```python
from build123d import *
from OCP.BRepFilletAPI import BRepFilletAPI_MakeChamfer

# Parameters (mm, degrees)
BOSS_EXTRUDE1_DEPTH = 20
SKETCH4_W           = 1
SKETCH4_H           = 9
CUT_EXTRUDE2_DEPTH  = 20
CUT_EXTRUDE4_START  = -2
CUT_EXTRUDE4_DEPTH  = 2
SKETCH5_R           = 2.6
CUT_EXTRUDE5_DEPTH  = 20
CHAMFER1_SIZE       = 0.4
CHAMFER1_SIZE2      = 0.406137053
CHAMFER1_SIZE2_2    = 0.394133002


with BuildPart() as part:
    # Sketch1 → Boss-Extrude1 (new body)
    with BuildSketch(Plane(origin=(0, 0, 0), x_dir=(1, 0, 0), z_dir=(0, 1, 0))):
        with BuildLine():
            Line((0, 9), (20, 9))
            Line((20, 9), (20, -9))
            Line((20, -9), (0, -9))
            ThreePointArc((0, -9), (-9, 0), (0, 9))
        make_face()
    extrude(amount=BOSS_EXTRUDE1_DEPTH)

    # Sketch7 → Cut-Revolve1 (revolve, cut)
    with BuildSketch(Plane.XY, mode=Mode.PRIVATE) as cut_revolve1_sk:
        Polygon((0, 0), (-6.1, 0), (-5.8, 20), (0, 20), align=None)
    revolve(cut_revolve1_sk.sketch.rotate(Axis((0, 20, 0), (0, 1, 0)), 180), axis=Axis((0, 20, 0), (0, 1, 0)), mode=Mode.SUBTRACT)

    # Sketch4 → Cut-Extrude2 (cut)
    with BuildSketch(Plane(origin=(0, 20, 0), x_dir=(1, 0, 0), z_dir=(0, 1, 0))):
        with Locations((0, 4.5)):
            Rectangle(SKETCH4_W, SKETCH4_H)
    extrude(amount=-CUT_EXTRUDE2_DEPTH, mode=Mode.SUBTRACT)

    # Sketch6 → Cut-Extrude4 (cut)
    with BuildSketch(Plane(origin=(0, 0, -9), x_dir=(-1, 0, 0), z_dir=(0, 0, -1)).offset(CUT_EXTRUDE4_START)):
        Polygon((-20, 12), (-14, 15.464101615), (-14, 4.535898385), (-20, 8), align=None)
    extrude(amount=-CUT_EXTRUDE4_DEPTH, mode=Mode.SUBTRACT)

    # Sketch5 → Cut-Extrude5 (cut)
    with BuildSketch(Plane(origin=(0, 20, 0), x_dir=(1, 0, 0), z_dir=(0, 1, 0))):
        with Locations(Location((11, 0, 0), (0, 0, 270))):
            Circle(SKETCH5_R)
    extrude(amount=-CUT_EXTRUDE5_DEPTH, mode=Mode.SUBTRACT)

    # Chamfer1: one chamfer whose edges measure the first distance from different faces: ONE call of the kernel's chamfer builder (chamfer() names one face for all edges)
    chamfer1_edges_1 = [part.edges().sort_by_distance(p)[0] for p in [
        (0, 0, 6.1),
    ]]
    chamfer1_side_1 = [part.faces().sort_by_distance(p)[0] for p in [
        (8.32015875, 0, 0.063305036),
    ]]
    chamfer1_edges_2 = [part.edges().sort_by_distance(p)[0] for p in [
        (0.5, 0, -7.539736831),
        (10.25, 0, -9),
        (20, 0, 0),
        (10, 0, 9),
        (-0.5, 0, -7.53278702),
        (-8.996524423, 0, 0.250096581),
        (11, 0, -2.6),
        (0.5, 20, -7.389204043),
        (10.25, 20, -9),
        (20, 20, 0),
        (10, 20, 9),
        (-8.996524423, 20, 0.250096581),
        (-0.5, 20, -7.382254232),
        (11, 20, -2.6),
    ]]
    chamfer1_edges_3 = [part.edges().sort_by_distance(p)[0] for p in [
        (0, 20, 5.8),
    ]]
    chamfer1_side_3 = [part.faces().sort_by_distance(p)[0] for p in [
        (0, 10, 5.95),
    ]]
    chamfer1 = BRepFilletAPI_MakeChamfer(part.part.solid().wrapped)
    for e in chamfer1_edges_1:
        chamfer1.Add(CHAMFER1_SIZE, CHAMFER1_SIZE2, e.wrapped, chamfer1_side_1[0].wrapped)  # the first distance lies on this face
    for e in chamfer1_edges_2:
        chamfer1.Add(CHAMFER1_SIZE, e.wrapped)
    for e in chamfer1_edges_3:
        chamfer1.Add(CHAMFER1_SIZE, CHAMFER1_SIZE2_2, e.wrapped, chamfer1_side_3[0].wrapped)  # the first distance lies on this face
    add(Compound.cast(chamfer1.Shape()), mode=Mode.REPLACE)


solid = part.part
```
Geometry check sheet. Reference: the model listing, model coordinates, mm. A direction names the side the tool comes from. Coordinates: 2 decimals unless noted, no trailing zeros. Loops run counter-clockwise (first coordinate to the right, second up) from the corner with the lowest first, then second, coordinate; pieces in that order, holes last. Notation, with made-up numbers: (51, -22) -> (84, -22) arc R28 cw to (84, 15) -> close; hole circle Ø1 at (40, 18.25). An arc over 180 degrees is marked (long way). Put each result on its own line as item: value.
1) Tool access check on faces 4 (the conical face through (-0.255, 10.137, 5.942)), 5 (the flat face through (16, 10, -7)), 6 (the flat face through (-0.5, 10, -7)). Record the directions out of +Z, -Z, +X, -X, +Y, -Y that give a thin tool (end or side, any length) a straight path to the whole face; none if there is none.
Result set:
face 4: -Y
face 5: none
face 6: -Z, +Y, -Y
2) Gauge pin test, flat ends, axial feed: pin 1 Ø3.5 at (y, z) = (12, -7.5) entering from -X; pin 2 Ø4.5 at (x, z) = (11, 0) entering from +Y; pin 3 Ø6 at (y, z) = (4.5, -3.5) entering from -X. Record the tip position at first contact, or that the pin passes through.
Result set:
pin 1: stops at x = -6.92
pin 2: passes through
pin 3: stops at x = -8.99
3) Thickness scan on line 1 (X direction, y = 19.25, z = -0.5); line 2 (X direction, y = 8.75, z = 0); line 3 (Z direction, x = 8.75, y = 8.25). Record the ranges inside material, lowest first.
Result set:
line 1: x = -8.99 to -5.79, 5.79 to 8.45, 13.55 to 20
line 2: x = -9 to -5.97, 5.97 to 8.4, 13.6 to 20
line 3: z = -9 to -1.3, 1.3 to 9
4) Cross-section at B-B on y = 8.5. Record the boundary of the cut face in (x, z) (1 decimal).
Result set:
outline: (-0.5, -9) -> (-0.5, -6) arc R6 cw (long way) to (0.5, -6) -> (0.5, -9) -> (20, -9) -> (20, -7) -> (14, -7) -> (14, -5) -> (20, -5) -> (20, 9) -> (0, 9) arc R9 ccw to start; hole circle Ø5.2 at (11, 0)
5) Cross-section at A-A on x = 11. Record the boundary of the cut face in (y, z).
Result set:
outline: (0, -8.6) -> (0.4, -9) -> (19.6, -9) -> (20, -8.6) -> (20, -3) -> (19.6, -2.6) -> (0.4, -2.6) -> (0, -3) -> close; (0, 3) -> (0.4, 2.6) -> (19.6, 2.6) -> (20, 3) -> (20, 8.6) -> (19.6, 9) -> (0.4, 9) -> (0, 8.6) -> close
6) Release check for a two-part mould opening along X. For faces 1 (the cylindrical face through (-9, 10, 0)), 2 (the cylindrical face through (8.46, 10.13, -0.56)), 3 (the flat face through (20, 10, 0)) record: released by +X, released by -X, zero draft, split by the parting line, or undercut.
Result set:
face 1: released by -X
face 2: undercut
face 3: released by +X
7) Cross-section at D-D on z = -0.5. Count the separate pieces of the cut face and the enclosed holes in it, plus the area to 3 significant figures.
Result set:
separate pieces: 3
enclosed holes: 0
area: 240 mm^2
8) Cross-section at C-C on y = 5.75. Record the boundary of the cut face in (x, z), plus the area to 3 significant figures.
Result set:
outline: (-0.5, -8.99) -> (-0.5, -5.99) arc R6.01 cw (long way) to (0.5, -5.99) -> (0.5, -9) -> (20, -9) -> (20, 9) -> (0, 9) arc R9 ccw to start; hole circle Ø5.2 at (11, 0); hole (14, -7) -> (16.1, -7) -> (16.1, -5) -> (14, -5) -> close
area: 345 mm^2
